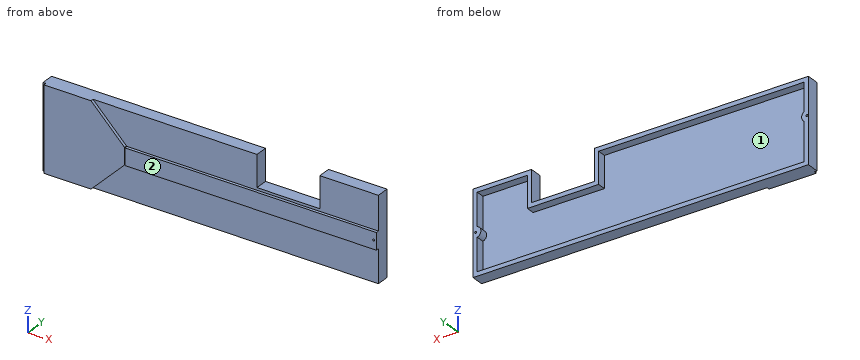
```python
from build123d import *

# Parameters (mm, degrees)
F0_R        = 0.635
F1_DEPTH    = 3.81
F2_T        = 2.54
F2_T3_DEPTH = 12.7
F3_W        = 152.4
F3_H        = 10.16
F3_R        = 0.635
F4_DEPTH    = 1.778
F5_W        = 48.9099100232
F5_H        = 50.8
F6_DEPTH    = 1.778
F7_SIZE     = 20.32


# Not quite as in the source:
# - a shell that OpenCascade refuses in one call is made with other operations: the cavity is built on its own and cut out


with BuildPart() as f1:
    # F0 (on Front) → F1 (new body, symmetric)
    with BuildSketch(Plane.XZ):
        Polygon((101.6, -25.4), (101.6, 25.4), (66.1107632279, 25.4), (66.1107632279, 6.35), (28.0107632279, 6.35), (28.0107632279, 25.4), (-101.6, 25.4), (-101.6, -25.4), align=None)
        with Locations((99.9609604478, 0)):
            Circle(F0_R, mode=Mode.SUBTRACT)
        with Locations((-100.653603673, 3.1339845154)):
            Circle(F0_R, mode=Mode.SUBTRACT)
    extrude(amount=F1_DEPTH, both=True)

    # F2: shell of thickness 2.54, made by hand


with BuildPart() as f2_core1:
    # F2_t2: copy of F1
    add(f1.part)

    # the walls: a layer under each face that stays
    f2_faces = [f2_core1.faces().sort_by_distance(p)[0] for p in [
        (101.6, 0, 0),
        (0, 0, -25.4),
        (-101.6, 0, 0),
        (-36.794618386, 0, 25.4),
        (28.0107632279, 0, 15.875),
        (47.0607632279, 0, 6.35),
        (66.1107632279, 0, 15.875),
        (0, -3.81, 0),
        (-101.288603673, 0, 3.1339845154),
        (99.3259604478, 0, 0),
        (83.855381614, 0, 25.4),
    ]]
    thicken(f2_faces, amount=-F2_T, mode=Mode.SUBTRACT)

    # F2_s4 → F2_t3 (cut)
    with BuildSketch(Plane.XZ.offset(-6.35)):
        Polygon((28.0361632279, 6.3754), (25.4707632279, 6.35), (25.4707632279, 3.81), (28.0107632279, 3.81), align=None)
        Polygon((66.0853632279, 6.3754), (66.1107632279, 3.81), (68.6507632279, 3.81), (68.6507632279, 6.35), align=None)
    extrude(amount=F2_T3_DEPTH, mode=Mode.SUBTRACT)


with BuildPart() as f1_1:
    add(f1.part)

    # what is left inside the walls is the cavity
    f2_cavity = [f2_core1.part.solids().sort_by_distance(p)[0] for p in [
        (0, 3.7846, -7.62),
    ]]
    add(f2_cavity, mode=Mode.SUBTRACT)

    # F3 (on face) → F4 (join)
    with BuildSketch(Plane.XZ.offset(3.81)):
        with Locations((25.4, -0.2157475356)):
            Rectangle(F3_W, F3_H)
        with Locations((99.9609604478, 0)):
            Circle(F3_R, mode=Mode.SUBTRACT)
    extrude(amount=F4_DEPTH)

    # F5 (on face) → F6 (join)
    with BuildSketch(Plane.XZ.offset(3.81)):
        with Locations((-75.4546709359, 0)):
            Rectangle(F5_W, F5_H)
    extrude(amount=F6_DEPTH)

    # F7
    f7_edges = [f1_1.edges().sort_by_distance(p)[0] for p in [
        (-50.999716, -4.699, 25.4),
        (-50.999716, -4.699, -25.4),
    ]]
    chamfer(f7_edges, length=F7_SIZE)


solid = f1_1.part
```
The model under review builds one solid part; all positions refer to its coordinate system, in mm. Face numbers are marked on the shaded views. Round coordinates to 2 decimals unless told otherwise and drop trailing zeros. Write each loop counter-clockwise with the first axis right and the second up, starting at its lowest first coordinate (ties: lowest second). Pieces come first, ordered by that corner, then holes. Notation, with made-up numbers: (12.5, -24.5) -> (53.5, -24.5) arc R25 ccw to (53.5, 7.5) -> close; hole circle Ø11 at (44, -6.75). An arc over 180 degrees is marked (long way). Use CSV: the item, a comma, the result in double quotes.
Q1. Consider section A-A (z = 11). Give the boundary of the cut face in (x, y), then the cut area to 3 significant figures.
Checks:
outline,"(-101.6, -3.81) -> (-99.91, -3.81) -> (-99.91, -5.59) -> (-56.92, -5.59) -> (-56.92, -3.81) -> (28.01, -3.81) -> (28.01, 3.81) -> (25.47, 3.81) -> (25.47, -1.27) -> (-99.06, -1.27) -> (-99.06, 3.81) -> (-101.6, 3.81) -> close; (66.11, -3.81) -> (101.6, -3.81) -> (101.6, 3.81) -> (99.06, 3.81) -> (99.06, -1.27) -> (68.65, -1.27) -> (68.65, 3.81) -> (66.11, 3.81) -> close"
area,"547 mm²"
Q2. Consider section D-D (x = -41.5). Give the boundary of the cut face in (y, z), then the cut area to 3 significant figures.
Checks:
outline,"(-5.59, -5.3) -> (-3.81, -5.3) -> (-3.81, -25.4) -> (3.81, -25.4) -> (3.81, -22.86) -> (-1.27, -22.86) -> (-1.27, 22.86) -> (3.81, 22.86) -> (3.81, 25.4) -> (-3.81, 25.4) -> (-3.81, 4.86) -> (-5.59, 4.86) -> close"
area,"173 mm²"
Q3. Consider section B-B (x = -86). Give the boundary of the cut face in (y, z).
Checks:
outline,"(-5.59, -25.4) -> (3.81, -25.4) -> (3.81, -22.86) -> (-1.27, -22.86) -> (-1.27, 22.86) -> (3.81, 22.86) -> (3.81, 25.4) -> (-5.59, 25.4) -> close"
Q4. Mouldability with a two-part tool opening along X and no side actions: class the marked faces 1 and 2 as released by +X, released by -X, zero draft, split by the parting line, or undercut.
Checks:
face 1,"undercut"
face 2,"zero draft"
Q5. Consider section C-C (x = 32.5). Give the boundary of the cut face in (y, z).
Checks:
outline,"(-5.59, -5.3) -> (-3.81, -5.3) -> (-3.81, -25.4) -> (3.81, -25.4) -> (3.81, -22.86) -> (-1.27, -22.86) -> (-1.27, 3.81) -> (3.81, 3.81) -> (3.81, 6.35) -> (-3.81, 6.35) -> (-3.81, 4.86) -> (-5.59, 4.86) -> close"
Q6. To check wall thickness, follow probe 1 along Z at (x, y) = (-51.5, 0.25); probe 2 along X at (y, z) = (1.5, 19); probe 3 along Z at (x, y) = (30, 3.25). State the ranges of each line that lie inside material, in increasing order. Write a range as [from, to].
Checks:
probe 1,"[-25.4, -22.86], [22.86, 25.4]"
probe 2,"[-101.6, -99.06], [25.47, 28.01], [66.11, 68.65], [99.06, 101.6]"
probe 3,"[-25.4, -22.86], [3.81, 6.35]"
Q7. For pin 1 Ø0.5 at (y, z) = (-5, -10.5) entering from -X; pin 2 Ø10 at (x, z) = (-29.5, 14.5) entering from -Y; pin 3 Ø1.5 at (x, z) = (80.5, 1.5) entering from +Y; pin 4 Ø1 at (x, z) = (-100.65, 3.13) entering from -Y, all flat-tipped, find the tip position at first contact; note any pin that passes through.
Checks:
pin 1,"x = -99.91"
pin 2,"y = -3.81"
pin 3,"y = -1.27"
pin 4,"through"
